For this review, take the finished solid that the model builds, in its own axes (mm). Face numbers are marked on the shaded views. Give positions to 0.01 mm unless a question says otherwise; leave off trailing zeros. Order: outer loops, then holes, each group sorted by start corner. A loop starts at its lowest first (then second) coordinate and runs counter-clockwise, first axis right, second up. Notation, with made-up numbers: (31, 33) - (44, 33) arc R26 ccw to (44, 65) - close; hole circle Ø10 at (-34, -24). An arc over 180 degrees is marked (long way). Answer as a JSON object with one key per item and string values. Group by question number.
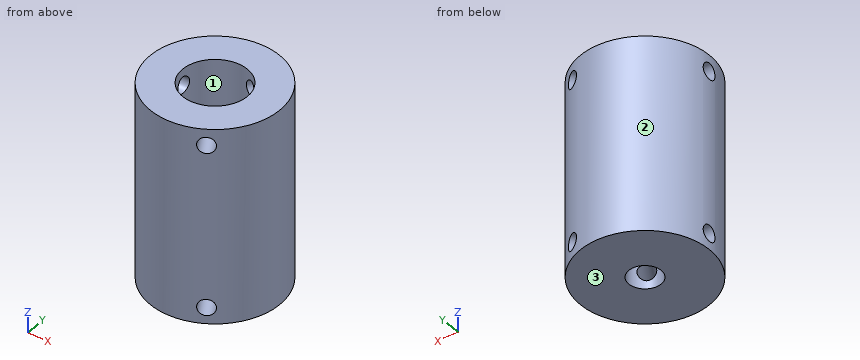
from build123d import *

# Parameters (mm, degrees)
SKETCH1_R           = 12.7
BOSS_EXTRUDE1_DEPTH = 19.05
SKETCH2_R           = 6.35
CUT_EXTRUDE1_DEPTH  = 19.05
SKETCH3_R           = 3.175
CUT_EXTRUDE2_DEPTH  = 19.05
SKETCH4_R           = 1.5875
CUT_EXTRUDE3_DEPTH  = 19.05
CIRPATTERN1_COUNT   = 3


with BuildPart() as part:
    # Sketch1 → Boss-Extrude1 (new, symmetric)
    with BuildSketch(Plane.XY):
        with Locations(Location((0, 0, 0), (0, 0, 180))):
            Circle(SKETCH1_R)
    extrude(amount=BOSS_EXTRUDE1_DEPTH, both=True)

    # Sketch2 → Cut-Extrude1 (cut)
    with BuildSketch(Plane.XY.offset(19.05)):
        Circle(SKETCH2_R)
    extrude(amount=-CUT_EXTRUDE1_DEPTH, mode=Mode.SUBTRACT)

    # Sketch3 → Cut-Extrude2 (cut)
    with BuildSketch(Plane(origin=(0, 0, -19.05), x_dir=(-1, 0, 0), z_dir=(0, 0, -1))):
        Circle(SKETCH3_R)
    extrude(amount=-CUT_EXTRUDE2_DEPTH, mode=Mode.SUBTRACT)

    # Sketch4 → Cut-Extrude3 (cut)
    with BuildSketch(Plane(origin=(0, 0, 0), x_dir=(0, 0, -1), z_dir=(1, 0, 0))):
        with Locations(Location((15.875, 0, 0), (0, 0, 180))):
            Circle(SKETCH4_R)
        with Locations((-15.875, 0)):
            Circle(SKETCH4_R)
    cut_extrude3 = extrude(amount=-CUT_EXTRUDE3_DEPTH, mode=Mode.SUBTRACT)

    # CirPattern1: Cut-Extrude3 ×3 about axis
    cirpattern1_axis = Axis((0, 0, 19.05), (0, 0, -1))
    for i in range(1, CIRPATTERN1_COUNT):
        add(cut_extrude3.rotate(cirpattern1_axis, i * 360 / CIRPATTERN1_COUNT), mode=Mode.SUBTRACT)


solid = part.part
1) Consider section A-A (y = 0). Give the number of separate pieces and of enclosed holes in the cut face, plus the area to 3 significant figures.
2) Consider section B-B (z = -15.5). Give the boundary of the cut face in (x, y) (3 decimals), plus the area to 3 significant figures.
3) Mouldability with a two-part tool opening along X and no side actions: class the marked faces 1, 2 and 3 as released by +X, released by -X, zero draft, split by the parting line, or undercut.
4) For line 1 (Y direction, x = 0, z = 14.5); line 2 (Z direction, x = -9, y = -0.5); line 3 (X direction, y = 0.25, z = -3), list the stretches that pass through material, from the lowest coordinate up.
5) Consider section D-D (x = -1.25). Give the boundary of the cut face in (y, z), plus the area to 3 significant figures.
6) For pin 1 (2 mm diameter, centred on x = -2, z = -6, fed in from +Y); pin 2 (10 mm diameter, centred on y = -8, z = -0.5, fed in from -X); pin 3 (1.5 mm diameter, centred on x = 8, z = -12.5, fed in from +Y), all flat-tipped, find the tip position at first contact; note any pin that passes through.
Result set:
{
 "1": {"separate pieces": "4", "enclosed holes": "0", "area": "554 mm2"},
 "2": {"outline": "(-12.606, -1.543) arc R12.7 ccw to (4.967, -11.688) - (0.052, -3.175) arc R3.175 cw to (-2.775, -1.543) - close; (-12.606, 1.543) - (-2.775, 1.543) arc R3.175 cw to (0.052, 3.175) - (4.967, 11.688) arc R12.7 ccw to start; (2.723, -1.632) - (7.639, -10.146) arc R12.7 ccw to (7.639, 10.146) - (2.723, 1.632) arc R3.175 cw to start", "area": "386 mm2"},
 "3": {"face 1": "undercut", "face 2": "split by the parting line", "face 3": "zero draft"},
 "4": {"line 1": "y = -12.7 to -6.35, 6.35 to 12.7", "line 2": "z = -19.05 to -17.38, -14.37 to 14.37, 17.38 to 19.05", "line 3": "x = -12.7 to -3.17, 3.17 to 12.7"},
 "5": {"outline": "(-12.64, -19.05) - (-2.92, -19.05) - (-2.92, 0) - (-6.23, 0) - (-6.23, 19.05) - (-12.64, 19.05) - close; (2.92, -19.05) - (12.64, -19.05) - (12.64, 19.05) - (6.23, 19.05) - (6.23, 0) - (2.92, 0) - close", "area": "615 mm2"},
 "6": {"pin 1": "stops at y = 12.66", "pin 2": "stops at x = -12.34", "pin 3": "stops at y = 10.43"}
}
